Geometry check sheet. Reference: drawing and pictorial views, mm from the part's lowest x, y, z. Round coordinates to 2 decimals unless told otherwise and drop trailing zeros. Order: outer loops, then holes, each group sorted by start corner. A loop starts at its lowest first (then second) coordinate and runs counter-clockwise, first axis right, second up.
(1) Thickness scan on probe 1 along Y at (x, z) = (38.5, 0.45); probe 2 along Y at (x, z) = (60.96, 2.45); probe 3 along X at (y, z) = (17, 1). Record the ranges inside material, lowest first.
(2) Sectioned sample at B-B, the plane y = 16.5. Enter the section's corners in (x, z).
(3) Sectioned sample at A-A, the plane x = 38.1. Enter the section's corners in (y, z).
(4) Sectioned sample at D-D, the plane x = 15.24. Enter the section's corners in (y, z).
(5) Depth check by flat-ended pin: pin 1 (8 mm diameter, centred on x = 62, y = 16.5, fed in from +Z); pin 2 (1.5 mm diameter, centred on x = 14, z = 2, fed in from -Y); pin 3 (1.5 mm diameter, centred on x = 2, z = 1, fed in from +Y); pin 4 (1.5 mm diameter, centred on y = 1, z = 1.5, fed in from -X). Enter the tip coordinate at first touch or a pass-through.
(6) Sectioned sample at C-C, the plane z = 0.6. Enter the section's corners in (x, y) (1 decimal).
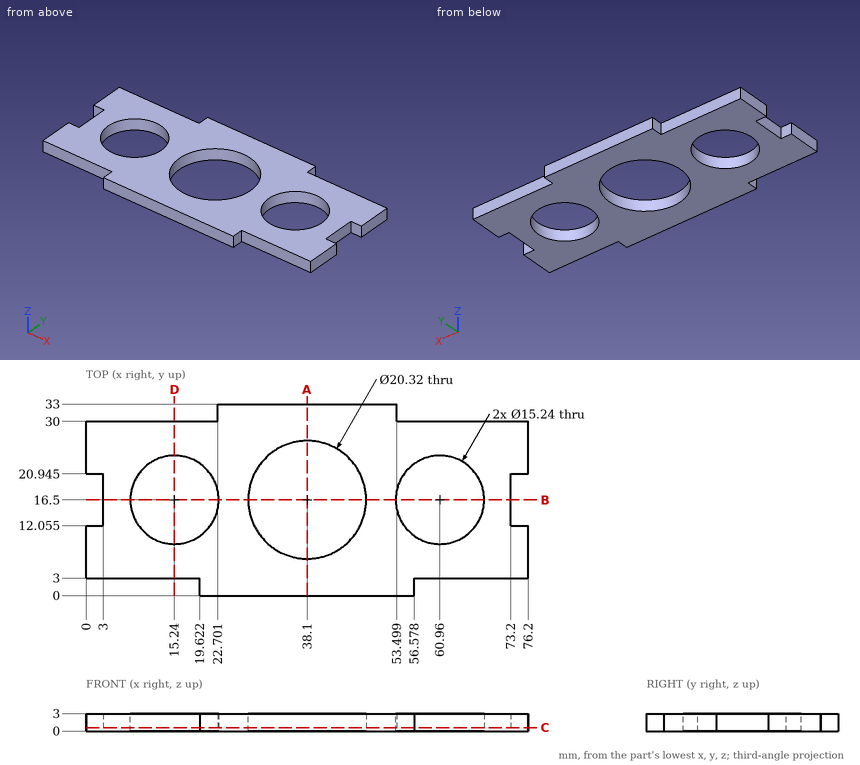
Derived:
1. probe 1: y = 0 to 6.35, 26.65 to 33
1. probe 2: y = 3 to 8.88, 24.12 to 30
1. probe 3: x = 3 to 7.64, 22.84 to 27.95, 48.25 to 53.36, 68.56 to 73.2
2. outline: (3, 0) - (7.62, 0) - (7.62, 3) - (3, 3) - close; (22.86, 0) - (27.94, 0) - (27.94, 3) - (22.86, 3) - close; (48.26, 0) - (53.34, 0) - (53.34, 3) - (48.26, 3) - close; (68.58, 0) - (73.2, 0) - (73.2, 3) - (68.58, 3) - close
3. outline: (0, 0) - (6.34, 0) - (6.34, 3) - (0, 3) - close; (26.66, 0) - (33, 0) - (33, 3) - (26.66, 3) - close
4. outline: (3, 0) - (8.88, 0) - (8.88, 3) - (3, 3) - close; (24.12, 0) - (30, 0) - (30, 3) - (24.12, 3) - close
5. pin 1: passes through
5. pin 2: stops at y = 3
5. pin 3: stops at y = 30
5. pin 4: stops at x = 19.62
6. outline: (0, 3) - (19.6, 3) - (19.6, 0) - (56.6, 0) - (56.6, 3) - (76.2, 3) - (76.2, 12.1) - (73.2, 12.1) - (73.2, 20.9) - (76.2, 20.9) - (76.2, 30) - (53.5, 30) - (53.5, 33) - (22.7, 33) - (22.7, 30) - (0, 30) - (0, 20.9) - (3, 20.9) - (3, 12.1) - (0, 12.1) - close; hole circle Ø15.2 at (15.2, 16.5); hole circle Ø20.3 at (38.1, 16.5); hole circle Ø15.2 at (61, 16.5)
